```python
from build123d import *

# Parameters (mm, degrees)
BOSS_EXTRU_1_DEPTH                             = 10
ESQUISSE2_R                                    = 1.5
ENL_V_MAT_EXTRU_1_DEPTH                        = 5
ESQUISSE3_R                                    = 1.5
ENL_V_MAT_EXTRU_2_DEPTH                        = 3
D_GAGEMENT_M31_D                               = 3.4
D_GAGEMENT_M31_DEPTH                           = 5
D_GAGEMENT_M31_TIP                             = 1.021463052
FRAISAGE_POUR_VIS_T_TE_FRAIS_E_M31_D           = 3.4
FRAISAGE_POUR_VIS_T_TE_FRAIS_E_M31_DEPTH       = 3
FRAISAGE_POUR_VIS_T_TE_FRAIS_E_M31_CSINK_D     = 6.3
FRAISAGE_POUR_VIS_T_TE_FRAIS_E_M31_CSINK_ANGLE = 90
FRAISAGE_POUR_VIS_T_TE_FRAIS_E_M31_TIP         = 1.021463052
CONG_1_R                                       = 3


with BuildPart() as part:
    # Esquisse1 → Boss.-Extru.1 (new body)
    with BuildSketch(Plane.XY):
        Polygon((15, 0), (15, 10), (10, 10), (10, 3), (0, 3), (0, 0), (10, 0), (10, -2.5), (15, -2.5), align=None)
    extrude(amount=BOSS_EXTRU_1_DEPTH)

    # Esquisse2 → Enlèv. mat.-Extru.1 (cut)
    with BuildSketch(Plane(origin=(15, 0, 0), x_dir=(0, 0, -1), z_dir=(1, 0, 0))):
        with Locations((-5, 6.5)):
            Circle(ESQUISSE2_R)
    extrude(amount=-ENL_V_MAT_EXTRU_1_DEPTH, mode=Mode.SUBTRACT)

    # Esquisse3 → Enlèv. mat.-Extru.2 (cut)
    with BuildSketch(Plane(origin=(0, 3, 0), x_dir=(1, 0, 0), z_dir=(0, 1, 0))):
        with Locations(Location((3.5, -5, 0), (0, 0, 180))):
            Circle(ESQUISSE3_R)
    extrude(amount=-ENL_V_MAT_EXTRU_2_DEPTH, mode=Mode.SUBTRACT)

    # Dégagement M31
    with Locations(Plane(origin=(15, 0, 0), x_dir=(0, 0, -1), z_dir=(1, 0, 0))):
        with Locations((-5, 6.5)):
            Hole(D_GAGEMENT_M31_D / 2, depth=D_GAGEMENT_M31_DEPTH)
            with Locations((0, 0, -(D_GAGEMENT_M31_DEPTH + D_GAGEMENT_M31_TIP / 2))):  # 118° drill point
                Cone(0, D_GAGEMENT_M31_D / 2, D_GAGEMENT_M31_TIP, mode=Mode.SUBTRACT)

    # Fraisage pour vis à tête fraisée M31
    with Locations(Plane(origin=(0, 3, 0), x_dir=(1, 0, 0), z_dir=(0, 1, 0))):
        with Locations((3.5, -5)):
            CounterSinkHole(FRAISAGE_POUR_VIS_T_TE_FRAIS_E_M31_D / 2, FRAISAGE_POUR_VIS_T_TE_FRAIS_E_M31_CSINK_D / 2, depth=FRAISAGE_POUR_VIS_T_TE_FRAIS_E_M31_DEPTH, counter_sink_angle=FRAISAGE_POUR_VIS_T_TE_FRAIS_E_M31_CSINK_ANGLE)
            with Locations((0, 0, -(FRAISAGE_POUR_VIS_T_TE_FRAIS_E_M31_DEPTH + FRAISAGE_POUR_VIS_T_TE_FRAIS_E_M31_TIP / 2))):  # 118° drill point
                Cone(0, FRAISAGE_POUR_VIS_T_TE_FRAIS_E_M31_D / 2, FRAISAGE_POUR_VIS_T_TE_FRAIS_E_M31_TIP, mode=Mode.SUBTRACT)

    # Congé1
    # the kernel refuses this fillet: 3 mm, written as the material it takes off along each edge
    with BuildSketch(Plane(origin=(0, 10.5, 10), x_dir=(0, 0, -1), z_dir=(0, -1, 0))) as cong_1_piece_1:
        with BuildLine():
            CenterArc((CONG_1_R, CONG_1_R), CONG_1_R, 180, 90)
            Line((0, CONG_1_R), (0, 0))
            Line((0, 0), (CONG_1_R, 0))
        make_face()
    extrude(amount=18, mode=Mode.SUBTRACT)
    with BuildSketch(Plane(origin=(0, 10.5, 0), x_dir=(0, 0, 1), z_dir=(0, -1, 0))) as cong_1_piece_2:
        with BuildLine():
            CenterArc((CONG_1_R, -CONG_1_R), CONG_1_R, 90, 90)
            Line((0, -CONG_1_R), (0, 0))
            Line((0, 0), (CONG_1_R, 0))
        make_face()
    extrude(amount=18, mode=Mode.SUBTRACT)
    with BuildSketch(Plane(origin=(22.5, 10, 0), x_dir=(0, -1, 0), z_dir=(-1, 0, 0)), Plane(origin=(2.5, -2.5, 10), x_dir=(0, 0, -1), z_dir=(1, 0, 0))) as cong_1_piece_3:
        with BuildLine():
            CenterArc((CONG_1_R, CONG_1_R), CONG_1_R, 180, 90)
            Line((0, CONG_1_R), (0, 0))
            Line((0, 0), (CONG_1_R, 0))
        make_face()
    extrude(amount=20, mode=Mode.SUBTRACT)
    with BuildSketch(Plane(origin=(22.5, 10, 10), x_dir=(0, -1, 0), z_dir=(-1, 0, 0)), Plane(origin=(2.5, -2.5, 0), x_dir=(0, 0, 1), z_dir=(1, 0, 0))) as cong_1_piece_4:
        with BuildLine():
            CenterArc((CONG_1_R, -CONG_1_R), CONG_1_R, 90, 90)
            Line((0, -CONG_1_R), (0, 0))
            Line((0, 0), (CONG_1_R, 0))
        make_face()
    extrude(amount=20, mode=Mode.SUBTRACT)


solid = part.part
```
Design review of the part built by this model. Coordinates are the model's own, in mm. A direction names the side the tool comes from. Round coordinates to 2 decimals unless told otherwise and drop trailing zeros. Order: outer loops, then holes, each group sorted by start corner. A loop starts at its lowest first (then second) coordinate and runs counter-clockwise, first axis right, second up. Notation, with made-up numbers: (37.5, 83) - (56.5, 83) arc R20 cw to (56.5, 106) - close; hole circle Ø7 at (30.5, -5.75). An arc over 180 degrees is marked (long way). Return JSON: item names as keys, results as strings.
Q1. Consider section D-D on x = 12. Write out the cut boundary in (y, z), plus the area to 3 significant figures.
Computed values:
{"outline": "(-2.5, 3) arc R3 ccw to (0.5, 0) - (7, 0) arc R3 ccw to (10, 3) - (10, 7) arc R3 ccw to (7, 10) - (0.5, 10) arc R3 ccw to (-2.5, 7) - close; hole circle Ø3.4 at (6.5, 5)", "area": "108 mm2"}
Q2. The part is to be moulded in two halves that separate along Z. For faces 1 (the cylindrical face through (12.5, 5, 5.8)), 2 (the flat face through (7, 3, 5)), 3 (the flat face through (10.2, 3.1, 10)), 4 (the flat face through (10.2, 3.1, 0)), say which applies: pulls with the +Z half, pulls with the -Z half, needs draft (parallel to the pull), parting line crosses it, or undercut.
Computed values:
{"face 1": "undercut", "face 2": "needs draft", "face 3": "pulls with the +Z half", "face 4": "pulls with the -Z half"}
Q3. Consider section B-B on x = 3.5. Write out the cut boundary in (y, z), plus the area to 3 significant figures.
Computed values:
{"outline": "(0, 0.04) arc R3 ccw to (0.5, 0) - (3, 0) - (3, 1.85) - (1.55, 3.3) - (0, 3.3) - close; (0, 6.7) - (1.55, 6.7) - (3, 8.15) - (3, 10) - (0.5, 10) arc R3 ccw to (0, 9.96) - close", "area": "17.7 mm2"}
Q4. Wall thickness on L1, parallel to Z at x = 3.5, y = 0.8; L2, parallel to Y at x = 13.2, z = 5; L3, parallel to Y at x = 9.5, z = 7.25: over which ranges is each line inside the solid? List them lowest first. Write a range as [from, to].
Computed values:
{"L1": "z = [0, 3.3], [6.7, 10]", "L2": "y = [-2.5, 4.8], [8.2, 10]", "L3": "y = [0, 3]"}
Q5. Consider section C-C on y = 6.5. Write out the cut boundary in (x, z), plus the area to 3 significant figures.
Computed values:
{"outline": "(10, 0) - (15, 0) - (15, 3.3) - (10, 3.3) - close; (10, 6.7) - (15, 6.7) - (15, 10) - (10, 10) - close", "area": "33.0 mm2"}
Q6. Consider section A-A on z = 5. Write out the cut boundary in (x, y).
Computed values:
{"outline": "(0, 0) - (1.8, 0) - (1.8, 1.55) - (0.35, 3) - (0, 3) - close; (5.2, 0) - (10, 0) - (10, -2.5) - (15, -2.5) - (15, 4.8) - (10, 4.8) - (10, 3) - (6.65, 3) - (5.2, 1.55) - close; (10, 8.2) - (15, 8.2) - (15, 10) - (10, 10) - close"}
Q7. Machinability: for faces 5 (the flat face through (10, 5, 3.8)), 6 (the cylindrical face through (11.44, -1.19, 9.48)), 7 (the flat face through (6, 0, 5)), which of the approach directions +Z, -Z, +X, -X, +Y, -Y give a long, thin tool a straight path to every point of the face, cutting with its end or side? Answer none if there is none.
Computed values:
{"face 5": "+Z, -Z, -X, +Y", "face 6": "+Z, +X, -X, -Y", "face 7": "+Z, -Z, -X, -Y"}
Q8. For pin 1 Ø5 at (x, z) = (3.5, 3.5) entering from +Y; pin 2 Ø4 at (x, y) = (12.5, 3.5) entering from -Z; pin 3 Ø3 at (x, z) = (3.5, 5) entering from +Y; pin 4 Ø3 at (x, z) = (3.5, 6) entering from -Y, all flat-tipped, find the tip position at first contact; note any pin that passes through.
Computed values:
{"pin 1": "stops at y = 3", "pin 2": "stops at z = 0", "pin 3": "passes through", "pin 4": "stops at y = 0"}
